Geometry: see drawing. Coordinates: mm, zero at the bounding-box minimum. A direction names the side the tool comes from. Coordinates: 2 decimals unless noted, no trailing zeros. Order: outer loops, then holes, each group sorted by start corner. A loop starts at its lowest first (then second) coordinate and runs counter-clockwise, first axis right, second up. Notation, with made-up numbers: (77.25, 29) -> (131.25, 29) arc R22 ccw to (131.25, 45) -> close; hole circle Ø1 at (-13, -40). An arc over 180 degrees is marked (long way). One line per item, written item: value. Start each with the question number.
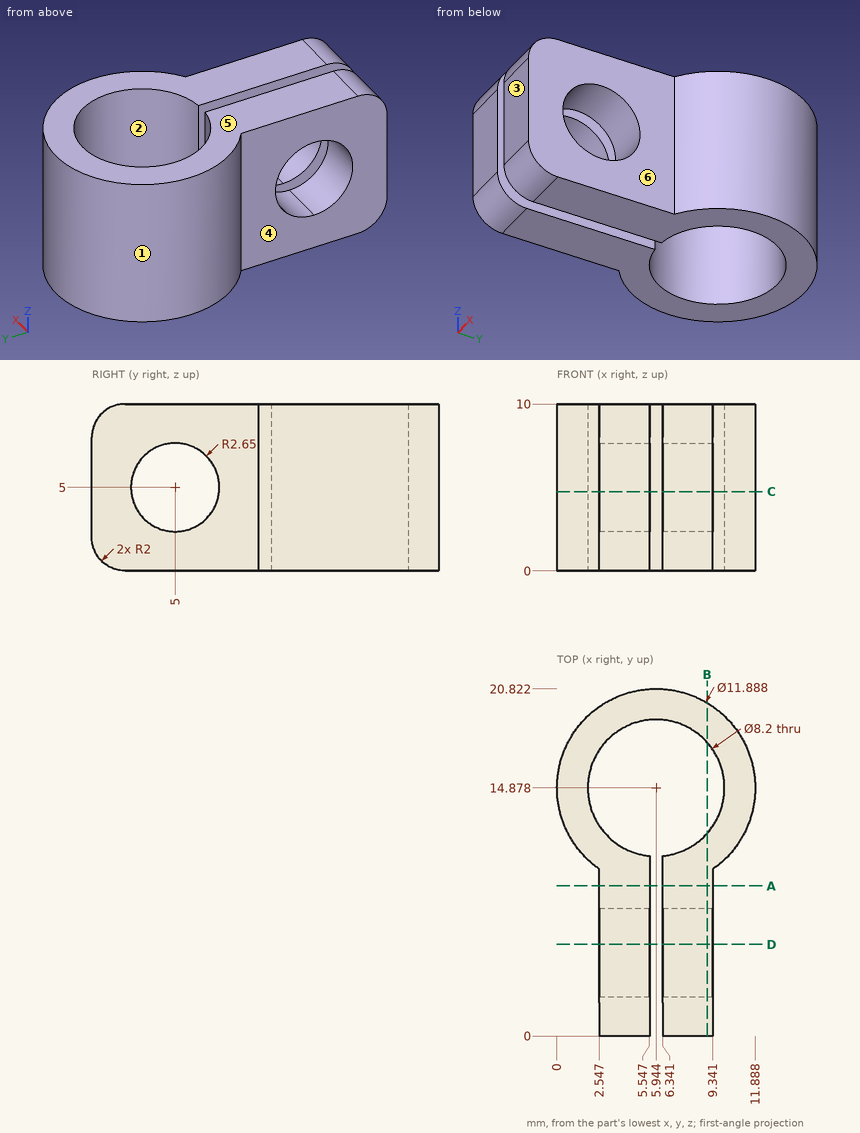
1) Pin query (flat end, axial travel): pin 1 Ø2 at (x, z) = (9, 7.5) entering from +Y (1 decimal); pin 2 Ø1.5 at (x, z) = (1.5, 6) entering from -Y; pin 3 Ø5 at (y, z) = (5.5, 6) entering from -X. Return the tip coordinate at first contact, or that it passes through.
2) Section query A-A, the plane y = 9. Return the cut outline in (x, z), plus the area to 3 significant figures.
3) Access query for the marked faces 4, 5 and 6. Directions: +Z, -Z, +X, -X, +Y, -Y. A direction counts if a zero-diameter tool reaches every point of the face in a straight line with its end or side. Return the directions, or none.
4) Ray query, line 1 along X through (y, z) = (7.5, 4); line 2 along Y through (x, z) = (7, 3.75) (1 decimal); line 3 along Y through (x, z) = (3, 6.75) (1 decimal). Return the intervals inside material, ascending. Write a range as from..to.
5) Section query B-B, the plane x = 9. State how many separate pieces and enclosed holes the cut face has, plus the area to 3 significant figures.
6) Mould query, pull axis X, two halves, no side actions, for the marked faces 1, 2 and 3. Classes: +X half, -X half, draft (parallel to the pull), parting line (faces both ways), or undercut.
7) Section query D-D, the plane y = 5.5. Return the cut outline in (x, z).
8) Section query C-C, the plane z = 4.75. Return the cut outline in (x, y).
Entries:
1. pin 1: stops at y = 20.5
1. pin 2: stops at y = 10.22
1. pin 3: stops at x = 2.55
2. outline: (2.55, 0) -> (5.55, 0) -> (5.55, 10) -> (2.55, 10) -> close; (6.34, 0) -> (9.34, 0) -> (9.34, 10) -> (6.34, 10) -> close
2. area: 60.0 mm2
3. face 4: +Z, -Z, -X, -Y
3. face 5: +Z, +X, -X, +Y, -Y
3. face 6: +Z, -Z, +X, -Y
4. line 1: x = 2.55..5.55, 6.34..9.34
4. line 2: y = 0..2.7, 7.3..10.9, 18.8..20.7
4. line 3: y = 0..3, 7..12, 17.7..20
5. separate pieces: 2
5. enclosed holes: 1
5. area: 121 mm2
6. face 1: parting line
6. face 2: undercut
6. face 3: draft
7. outline: (2.55, 0) -> (5.55, 0) -> (5.55, 2.4) -> (2.55, 2.4) -> close; (2.55, 7.6) -> (5.55, 7.6) -> (5.55, 10) -> (2.55, 10) -> close; (6.34, 0) -> (9.34, 0) -> (9.34, 2.4) -> (6.34, 2.4) -> close; (6.34, 7.6) -> (9.34, 7.6) -> (9.34, 10) -> (6.34, 10) -> close
8. outline: (2.55, 0) -> (5.55, 0) -> (5.55, 2.36) -> (2.55, 2.36) -> close; (2.55, 7.64) -> (5.55, 7.64) -> (5.55, 10.8) arc R4.1 cw (long way) to (6.34, 10.8) -> (6.34, 7.64) -> (9.34, 7.64) -> (9.34, 10) arc R5.94 ccw (long way) to (2.55, 10) -> close; (6.34, 0) -> (9.34, 0) -> (9.34, 2.36) -> (6.34, 2.36) -> close
